```python
from build123d import *

# Parameters (mm, degrees)
F0_R     = 522.5
F1_DEPTH = 3.18


with BuildPart() as f1:
    # F0 (on Top) → F1 (new body)
    with BuildSketch(Plane.XY):
        Circle(F0_R)
        with BuildLine():
            ThreePointArc((385.144778, 257.95756), (443.515763, 134.804935), (463.55, 0))
            ThreePointArc((463.55, 0), (461.337407, -45.237144), (454.720751, -90.04244))
            ThreePointArc((454.720751, -90.04244), (454.115986, -93.04447), (453.491403, -96.04244))
            ThreePointArc((453.491403, -96.04244), (293.018375, -359.191919), (3, -463.540292))
            ThreePointArc((3, -463.540292), (0, -463.55), (-3, -463.540292))
            ThreePointArc((-3, -463.540292), (-210.136781, -413.184142), (-372.83495, -275.45))
            ThreePointArc((-372.83495, -275.45), (-375.026465, -272.458718), (-377.193982, -269.45))
            ThreePointArc((-377.193982, -269.45), (-451.864779, -103.42545), (-456.846254, 78.55))
            ThreePointArc((-456.846254, 78.55), (-456.319967, 81.551762), (-455.773957, 84.55))
            ThreePointArc((-455.773957, 84.55), (-97.171992, 453.25071), (381.05775, 263.95756))
            ThreePointArc((381.05775, 263.95756), (383.11301, 260.965561), (385.144778, 257.95756))
        make_face(mode=Mode.SUBTRACT)
        with BuildLine():
            Line((-3, 84.55), (-455.773957, 84.55))
            ThreePointArc((-455.773957, 84.55), (-456.319967, 81.551762), (-456.846254, 78.55))
            Line((-456.846254, 78.55), (-3, 78.55))
            Line((-3, 78.55), (-3, 84.55))
        make_face()
        with BuildLine():
            Line((3, 257.95756), (385.144778, 257.95756))
            ThreePointArc((385.144778, 257.95756), (383.11301, 260.965561), (381.05775, 263.95756))
            Line((381.05775, 263.95756), (-3, 263.95756))
            Line((-3, 263.95756), (-3, 84.55))
            Line((-3, 84.55), (-3, 78.55))
            Line((-3, 78.55), (-3, -269.45))
            Line((-3, -269.45), (-3, -275.45))
            Line((-3, -275.45), (-3, -463.540292))
            ThreePointArc((-3, -463.540292), (0, -463.55), (3, -463.540292))
            Line((3, -463.540292), (3, -96.04244))
            Line((3, -96.04244), (3, -90.04244))
            Line((3, -90.04244), (3, 257.95756))
        make_face()
        with BuildLine():
            ThreePointArc((453.491403, -96.04244), (454.115986, -93.04447), (454.720751, -90.04244))
            Line((454.720751, -90.04244), (3, -90.04244))
            Line((3, -90.04244), (3, -96.04244))
            Line((3, -96.04244), (453.491403, -96.04244))
        make_face()
        with BuildLine():
            Line((-3, -269.45), (-377.193982, -269.45))
            ThreePointArc((-377.193982, -269.45), (-375.026465, -272.458718), (-372.83495, -275.45))
            Line((-372.83495, -275.45), (-3, -275.45))
            Line((-3, -275.45), (-3, -269.45))
        make_face()
    extrude(amount=F1_DEPTH)


solid = f1.part
```
Can you work these out from the model? Positions are in its coordinate system, mm. A direction names the side the tool comes from. Round coordinates to 2 decimals unless told otherwise and drop trailing zeros. Loops run counter-clockwise (first coordinate to the right, second up) from the corner with the lowest first, then second, coordinate; pieces in that order, holes last.
Item 1: Will these pins go through, and if not, where does the flat tip stop? pin 1 Ø1 at (x, z) = (227, 1) entering from -Y; pin 2 Ø1 at (x, z) = (171.5, 1) entering from +Y; pin 3 Ø1 at (x, z) = (-226, 1) entering from +Y.
Item 2: Suppose I cut it at B-B, the plane x = -361. Write out the boundary of the cut face in (y, z), then the cut area to 3 significant figures.
Item 3: Please list where these lines run through material, in increasing order: L1, parallel to X at y = -1, z = 1.75; L2, parallel to X at y = -32.5, z = 1.6; L3, parallel to Y at x = -45, z = 2.75.
Item 4: If we mould it in two halves opening along X, with no side actions, what happens to faces 1 (the flat face through (-2, -36, 3.18)), 2 (the cylindrical face through (442.955, 136.636, 1.568)), 3 (the cylindrical face through (498.372, 156.945, 1.568))? For each: +X half, -X half, draft (parallel to the pull), parting line (faces both ways), or undercut.
Item 5: Suppose I cut it at C-C, the plane y = -230. Write out the boundary of the cut face in (x, z), then the cut area to 3 significant figures.
Item 6: Suppose I cut it at D-D, the plane x = 402.5. Write out the boundary of the cut face in (y, z), then the cut area to 3 significant figures.
Item 7: Suppose I cut it at A-A, the plane z = 1.4. Write out the boundary of the cut face in (x, y), then the cut area to 3 significant figures.
Item 8: Which directions (+Z, -Z, +X, -X, +Y, -Y) give clear straight access to the entire face, cutting with the end or side of a thin tool? Please do faces 4 (the flat face through (-2, -36, 0)), 5 (the cylindrical face through (-451.286, -105.924, 1.568)).
Reported:
1. pin 1: stops at y = -470.85
1. pin 2: stops at y = 493.73
1. pin 3: stops at y = 471.33
2. outline: (-377.74, 0) - (-290.79, 0) - (-290.79, 3.18) - (-377.74, 3.18) - close; (-275.45, 0) - (-269.45, 0) - (-269.45, 3.18) - (-275.45, 3.18) - close; (78.55, 0) - (84.55, 0) - (84.55, 3.18) - (78.55, 3.18) - close; (290.79, 0) - (377.74, 0) - (377.74, 3.18) - (290.79, 3.18) - close
2. area: 591 mm2
3. L1: x = -522.5 to -463.55, -3 to 3, 463.55 to 522.5
3. L2: x = -521.49 to -462.41, -3 to 3, 462.41 to 521.49
3. L3: y = -520.56 to -461.36, -275.45 to -269.45, 78.55 to 84.55, 461.36 to 520.56
4. face 1: draft
4. face 2: undercut
4. face 3: parting line
5. outline: (-469.15, 0) - (-402.47, 0) - (-402.47, 3.18) - (-469.15, 3.18) - close; (-3, 0) - (3, 0) - (3, 3.18) - (-3, 3.18) - close; (402.47, 0) - (469.15, 0) - (469.15, 3.18) - (402.47, 3.18) - close
5. area: 443 mm2
6. outline: (-333.17, 0) - (-229.94, 0) - (-229.94, 3.18) - (-333.17, 3.18) - close; (-96.04, 0) - (-90.04, 0) - (-90.04, 3.18) - (-96.04, 3.18) - close; (229.94, 0) - (333.17, 0) - (333.17, 3.18) - (229.94, 3.18) - close
6. area: 676 mm2
7. outline: circle Ø1045 at (0, 0); hole (-456.85, 78.55) arc R463.55 ccw to (-377.19, -269.45) - (-3, -269.45) - (-3, 78.55) - close; hole (-455.77, 84.55) - (-3, 84.55) - (-3, 263.96) - (381.06, 263.96) arc R463.55 ccw to start; hole (-372.83, -275.45) arc R463.55 ccw to (-3, -463.54) - (-3, -275.45) - close; hole (3, -463.54) arc R463.55 ccw to (453.49, -96.04) - (3, -96.04) - close; hole (3, -90.04) - (454.72, -90.04) arc R463.55 ccw to (463.55, 0) arc R463.55 ccw to (385.14, 257.96) - (3, 257.96) - close
7. area: 197,000 mm2
8. face 4: -Z, +X, -X, +Y, -Y
8. face 5: +Z, -Z
